Input: part model. Units: mm. Frame: model coordinates. Face numbers are marked on the shaded views. A direction names the side the tool comes from. Round coordinates to 2 decimals unless told otherwise and drop trailing zeros. Loops run counter-clockwise (first coordinate to the right, second up) from the corner with the lowest first, then second, coordinate; pieces in that order, holes last.
1) Section C-C, the plane x = -21. Return loops of the section in (y, z), and give its area (3 significant figures).
2) Ray query, line 1 along X through (y, z) = (-1.5, 14.5); line 2 along Z through (x, y) = (-23.5, -5.5); line 3 along Z through (x, y) = (-41, -1.25). Return the intervals inside material, ascending.
3) Section A-A, the plane y = -6.5. Return loops of the section in (x, z).
4) First-contact query: pin 1 (6 mm diameter, centred on x = -24.5, y = -10.5, fed in from +Z); pin 2 (6.5 mm diameter, centred on x = -38, y = -14.5, fed in from +Z); pin 3 (3.5 mm diameter, centred on y = -13.5, z = 19, fed in from -X). Flat tips, straight axial feed; report the tip coordinate or a pass-through.
5) Section B-B, the plane z = 27.5. Return loops of the section in (x, y), and give its area (3 significant figures).
6) Access query for the marked faces 1 and 2. Directions: +Z, -Z, +X, -X, +Y, -Y. A direction counts if a zero-diameter tool reaches every point of the face in a straight line with its end or side. Return the directions, or none.
from build123d import *

# Parameters (mm, degrees)
F0_W     = 8
F0_H     = 14
F1_DEPTH = 30


with BuildPart() as f1:
    # F0 (on Front) → F1 (new body)
    with BuildSketch(Plane.XZ):
        with Locations((-39, 7)):
            Rectangle(F0_W, F0_H)
        Polygon((-13, 0), (0, 0), (0, 43), (-13, 43), (-13, 33), align=None)
        Polygon((-25, 0), (-13, 0), (-13, 33), (-25, 33), (-25, 25), align=None)
        Polygon((-35, 0), (-25, 0), (-25, 25), (-35, 25), (-35, 14), align=None)
    extrude(amount=F1_DEPTH)


solid = f1.part
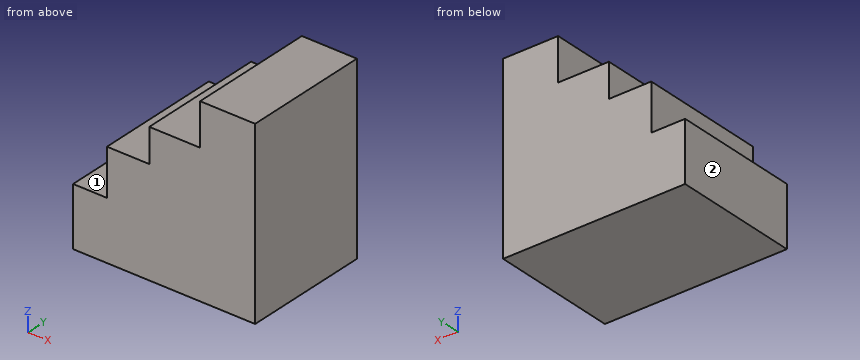
Final values:
1. outline: (-30, 0) - (0, 0) - (0, 33) - (-30, 33) - close
1. area: 990 mm2
2. line 1: x = -35 to 0
2. line 2: z = 0 to 33
2. line 3: z = 0 to 14
3. outline: (-43, 0) - (0, 0) - (0, 43) - (-13, 43) - (-13, 33) - (-25, 33) - (-25, 25) - (-35, 25) - (-35, 14) - (-43, 14) - close
4. pin 1: stops at z = 33
4. pin 2: stops at z = 25
4. pin 3: stops at x = -35
5. outline: (-25, -30) - (0, -30) - (0, 0) - (-25, 0) - close
5. area: 750 mm2
6. face 1: +Z, -X, +Y, -Y
6. face 2: +Z, -Z, -X, +Y, -Y
